For this review, take the finished solid that the model builds, in its own axes (mm). A direction names the side the tool comes from. Coordinates: 2 decimals unless noted, no trailing zeros. Loops run counter-clockwise (first coordinate to the right, second up) from the corner with the lowest first, then second, coordinate; pieces in that order, holes last. Notation, with made-up numbers: M 11.5,35.5 L 23.5,35.5 A25 ccw 23.5,61.5 Z; hole C 74.25,59.25 d11. An arc over 180 degrees is marked long. Write each question's results on one line, items separated by ' | '. Start each with the question number.
```python
from build123d import *

# Parameters (mm, degrees)
SKETCH1_W           = 214.089522673
SKETCH1_H           = 271.033566845
BOSS_EXTRUDE1_DEPTH = 10
SKETCH3_W           = 107.044761337
SKETCH3_H           = 271.033566845
CUT_EXTRUDE1_DEPTH  = 252.253590179
CUT_EXTRUDE2_DEPTH  = 249.55642867
BOSS_EXTRUDE3_DEPTH = 40
CUT_EXTRUDE3_START  = -165.689856025
CUT_EXTRUDE3_DEPTH  = 205.862728092
CUT_EXTRUDE4_DEPTH  = 250.960593361
CUT_EXTRUDE5_DEPTH  = 250.960593361
BOSS_EXTRUDE5_DEPTH = 45
CUT_EXTRUDE7_DEPTH  = 253.784190336
CUT_EXTRUDE9_DEPTH  = 253.784190336
CUT_EXTRUDE10_DEPTH = 253.784190336
BOSS_EXTRUDE6_DEPTH = 13.546139965


with BuildPart() as part:
    # Sketch1 → Boss-Extrude1 (new body)
    with BuildSketch(Plane(origin=(0, 0, 0), x_dir=(1, 0, 0), z_dir=(0, 1, 0))):
        with Locations((-3.148375333, -90.062114546)):
            Rectangle(SKETCH1_W, SKETCH1_H)
    extrude(amount=BOSS_EXTRUDE1_DEPTH)

    # Sketch3 → Cut-Extrude1 (cut, through all)
    with BuildSketch(Plane(origin=(0, 10, 0), x_dir=(1, 0, 0), z_dir=(0, 1, 0))):
        with Locations((-56.670756002, -90.062114546)):
            Rectangle(SKETCH3_W, SKETCH3_H)
    extrude(amount=-CUT_EXTRUDE1_DEPTH, mode=Mode.SUBTRACT)

    # Sketch4 → Cut-Extrude2 (cut, through all)
    with BuildSketch(Plane(origin=(0, 10, 0), x_dir=(1, 0, 0), z_dir=(0, 1, 0))):
        Polygon((103.896386003, -181.239506042), (100.834918545, -173.848469781), (9.996584241, 45.454668877), (103.896386003, 45.454668877), align=None)
    extrude(amount=-CUT_EXTRUDE2_DEPTH, mode=Mode.SUBTRACT)

    # Sketch6 → Boss-Extrude3 (add, along a direction that is not the sketch's normal)
    with BuildSketch(Plane(origin=(0, 10, 0), x_dir=(1, 0, 0), z_dir=(0, 1, 0))):
        Polygon((99.572063218, -170.799667324), (103.896386003, -181.239506042), (-3.148375333, -225.578897968), (-3.148375333, -213.347866105), align=None)
    extrude(amount=BOSS_EXTRUDE3_DEPTH, dir=(-0.2705980500730979, 0.7071067811865489, -0.6532814824381872))

    # Cut-Extrude3: read off the stored shape, not the designer's step
    # Cut-Extrude3 outline → Cut-Extrude3 (cut)
    with BuildSketch(Plane(origin=(0, 0, 0), x_dir=(1, 0, 0), z_dir=(0, 0.6785983445458481, -0.7345095552677544)).offset(CUT_EXTRUDE3_START)):
        Polygon((-3.148375333, -165), (-3.148375333, -152.122604304), (-13.972297336, -155.165042499), (-15, -155.45391393), (-15, -165), align=None)
    extrude(amount=CUT_EXTRUDE3_DEPTH, mode=Mode.SUBTRACT)

    # Sketch8 → Cut-Extrude4 (cut, through all)
    with BuildSketch(Plane(origin=(0, 10, 0), x_dir=(1, 0, 0), z_dir=(0, 1, 0))):
        Polygon((-3.148375333, -225.578897968), (103.896386003, -181.239506042), (103.896386003, -225.578897968), align=None)
    extrude(amount=-CUT_EXTRUDE4_DEPTH, mode=Mode.SUBTRACT)

    # Sketch9 → Cut-Extrude5 (cut, through all)
    with BuildSketch(Plane(origin=(0, 10, 0), x_dir=(1, 0, 0), z_dir=(0, 1, 0))):
        Polygon((-3.148375333, -213.347866105), (99.572063218, -170.799667324), (9.996584241, 45.454668877), (-3.148375333, 45.454668877), align=None)
    extrude(amount=-CUT_EXTRUDE5_DEPTH, mode=Mode.SUBTRACT)

    # Sketch13 → Boss-Extrude5 (add)
    with BuildSketch(Plane.XZ):
        Polygon((-3.148375333, 225.578897968), (-3.148375333, 213.347866105), (99.572063218, 170.799667324), (103.896386003, 181.239506042), align=None)
    extrude(amount=BOSS_EXTRUDE5_DEPTH)

    # Sketch14 → Cut-Extrude7 (cut, through all)
    with BuildSketch(Plane(origin=(24.603270673, 0, -10.191008392), x_dir=(-0.38268343236508967, 0, -0.9238795325112868), z_dir=(0.9238795325112867, 0, -0.3826834323650896))):
        Polygon((-178.918624473, 38.284271247), (-173.268624473, 32.634271247), (-167.618624473, 38.284271247), align=None)
    extrude(amount=-CUT_EXTRUDE7_DEPTH, mode=Mode.SUBTRACT)

    # Sketch21 → Cut-Extrude9 (cut, through all)
    with BuildSketch(Plane(origin=(24.603270673, 0, -10.191008392), x_dir=(-0.38268343236508967, 0, -0.9238795325112868), z_dir=(0.9238795325112867, 0, -0.3826834323650896))):
        Polygon((-178.918624473, 38.284271247), (-173.268624473, 32.634271247), (-186.710507565, 19.192388155), (-188.372208501, 20.854089091), (-197.564596656, 11.661700936), (-199.891194785, 13.988299064), (-190.698806629, 23.18068722), (-192.360507565, 24.842388155), align=None)
    extrude(amount=-CUT_EXTRUDE9_DEPTH, mode=Mode.SUBTRACT)

    # Sketch23 → Cut-Extrude10 (cut, through all)
    with BuildSketch(Plane(origin=(24.603270673, 0, -10.191008392), x_dir=(-0.38268343236508967, 0, -0.9238795325112868), z_dir=(0.9238795325112867, 0, -0.3826834323650896))):
        Polygon((-207.20289572, -3), (-203.20289572, -3), (-203.20289572, 10), (-199.90289572, 10), (-199.90289572, -3), (-195.90289572, -3), (-195.90289572, -45), (-207.20289572, -45), align=None)
    extrude(amount=-CUT_EXTRUDE10_DEPTH, mode=Mode.SUBTRACT)

    # Sketch24 → Boss-Extrude6 (add, along a direction that is not the sketch's normal)
    with BuildSketch(Plane(origin=(35.57097911, -92.95144786, 85.875940195), x_dir=(0.9626924198811571, 0.19875685341551327, -0.18362738881693624), z_dir=(-0.2705980500730966, 0.7071067811865525, -0.6532814824381838))):
        Polygon((-40.219860097, -165.940754997), (-40.219860097, -169.369289928), (-38.335322468, -168.817321636), (-39.260177115, -165.659670359), align=None)
    extrude(amount=BOSS_EXTRUDE6_DEPTH, dir=(0, 0.6785983445458494, -0.7345095552677533))


solid = part.part
```
Q1. Take a section at A-A, the plane y = 8. Give the boundary of the cut face in (x, z), then the cut area to 3 significant figures.
Q2. Insertion check: P1, Ø1.5, axis at x = 39.5, y = 2, coming from the +Z side; P2, Ø4, axis at x = 53, y = 6.5, coming from the +Z side; P3, Ø2, axis at x = 56, y = 17.5, coming from the -Z side; P4, Ø4, axis at x = 80.5, z = 185.5, coming from the -Y side. Each pin has a flat end and moves straight along its axis. Give the tip position at first contact, or say it passes through.
Q3. The part is to be moulded in two halves that separate along Z. For faces 1 (the face through (-1.773, 17.373, 210.948)), 2 (the face through (51.12, 3.59, 203.1)), 3 (the face through (47.493, 3.591, 192.372)), say which applies: pulls with the +Z half, pulls with the -Z half, needs draft (parallel to the pull), parting line crosses it, or undercut.
Q4. Take a section at D-D, the plane z = 183.5. Give the boundary of the cut face in (x, y), then the cut area to 3 significant figures.
Q5. For faces 4 (the face through (-3.148, 10, 216)), 5 (the face through (50, 10, 198)), 6 (the face through (47.93, 16.32, 188.95)), list the 3-axis set-ups (+Z, -Z, +X, -X, +Y, -Y) from which the entire face can be reached by the end or side of a thin tool; tool diameter is ignored.
Q6. To check wall thickness, follow line 1 along Z through (x, y) = (31, 0.5); line 2 along Z through (x, y) = (20, 13.5); line 3 along X through (y, z) = (1, 189.5). State the ranges of each line that lie inside material, in increasing order.
Q7. Take a section at B-B, the plane z = 169. Give the boundary of the cut face in (x, y).
Q8. Take a section at C-C, the plane x = 43.5. Give the boundary of the cut face in (y, z).
Results:
1) outline: M -3.15,213.35 L 99.57,170.8 L 101.1,174.5 L -3.15,217.68 Z; M -3.15,221.25 L 102.37,177.54 L 103.9,181.24 L -3.15,225.58 Z | area: 908 mm^2
2) P1: z = 208.22 | P2: z = 203.15 | P3: z = 179.57 | P4: y = -3
3) face 1: undercut | face 2: pulls with the +Z half | face 3: pulls with the -Z half
4) outline: M 44.89,19.19 L 68.91,10 L 68.91,-3 L 79.36,-3 L 79.36,10 L 87.99,10 L 87.99,-3 L 98.44,-3 L 98.44,10 L 59.65,24.84 L 55.31,23.18 L 79.33,13.99 L 73.25,11.66 L 49.23,20.85 Z | area: 515 mm^2
5) face 4: +Z, -Z, -X, +Y, -Y | face 5: -Y | face 6: none
6) line 1: 199.2 to 203.53, 207.1 to 211.43 | line 2: 199.97 to 203.57, 207.55 to 212.2 | line 3: 54.43 to 64.88, 73.5 to 83.95
7) outline: M 79.9,19.19 L 98.83,11.95 L 98.83,15.27 L 84.24,20.85 Z; M 90.32,23.18 L 98.83,19.92 L 98.83,23.25 L 94.66,24.84 Z
8) outline: M -3,194.03 L 10,194.03 L 19.19,184.08 L 20.85,185.87 L 11.66,195.82 L 13.99,198.34 L 23.18,188.39 L 24.84,190.19 L 10,206.26 L -3,206.26 L -3,201.93 L 10,201.93 L 10,198.36 L -3,198.36 Z
